```python
from build123d import *

# Parameters (mm, degrees)
ESBO_O1_R                                            = 10.7
RESSALTO_EXTRUS_O1_DEPTH                             = 2.05
RESSALTO_EXTRUS_O2_DEPTH                             = 3
ESBO_O4_W                                            = 25
ESBO_O4_H                                            = 7.35
RESSALTO_EXTRUS_O3_DEPTH                             = 10.8
REBAIXO_PARA_SHCS_M2_51_D                            = 2.9
REBAIXO_PARA_SHCS_M2_51_CBORE_D                      = 5.5
REBAIXO_PARA_SHCS_M2_51_CBORE_DEPTH                  = 10
REBAIXO_PARA_PARAFUSO_COM_CABE_A_REDONDA_D           = 2.4
REBAIXO_PARA_PARAFUSO_COM_CABE_A_REDONDA_CBORE_D     = 4.4
REBAIXO_PARA_PARAFUSO_COM_CABE_A_REDONDA_CBORE_DEPTH = 3.5
PADR_OCIRCULAR1_COUNT                                = 4
NERVURA1_REACH                                       = 67.842
ESBO_O5_WALL_W                                       = 144.857085312
ESBO_O5_WALL_H                                       = 15
CORTE_EXTRUS_O1_REACH                                = 68.053
ESBO_O6_W                                            = 8.93885445
ESBO_O6_H                                            = 8
CORTE_EXTRUS_O2_REACH                                = 68.474
ESBO_O7_R                                            = 3
FILETE1_R                                            = 2


with BuildPart() as part:
    # Esboço1 → Ressalto-extrusão1 (new body)
    with BuildSketch(Plane(origin=(0, 0, 0), x_dir=(-1, 0, 0), z_dir=(0, 0, -1))):
        Circle(ESBO_O1_R)
    extrude(amount=RESSALTO_EXTRUS_O1_DEPTH)

    # Esboço2 → Ressalto-extrusão2 (add)
    with BuildSketch(Plane(origin=(0, 0, -2.05), x_dir=(-1, 0, 0), z_dir=(0, 0, -1))):
        with BuildLine():
            Line((-12.5, 64.388275999), (12.5, 64.388275999))
            Line((12.5, 64.388275999), (12.5, 0))
            ThreePointArc((12.5, 0), (0, -12.5), (-12.5, 0))
            Line((-12.5, 0), (-12.5, 64.388275999))
        make_face()
    extrude(amount=RESSALTO_EXTRUS_O2_DEPTH)

    # Esboço4 → Ressalto-extrusão3 (add)
    with BuildSketch(Plane(origin=(0, 0, -5.05), x_dir=(-1, 0, 0), z_dir=(0, 0, -1))):
        with Locations((0, 60.713275999)):
            Rectangle(ESBO_O4_W, ESBO_O4_H)
    extrude(amount=-RESSALTO_EXTRUS_O3_DEPTH)

    # Rebaixo para SHCS M2.51 (through all)
    with Locations(Plane(origin=(0, 0, -5.05), x_dir=(-1, 0, 0), z_dir=(0, 0, -1))):
        with Locations((-8.5, 61.838275999), (8.5, 61.838275999)):
            CounterBoreHole(REBAIXO_PARA_SHCS_M2_51_D / 2, REBAIXO_PARA_SHCS_M2_51_CBORE_D / 2, REBAIXO_PARA_SHCS_M2_51_CBORE_DEPTH)

    # Rebaixo para parafuso com cabeça redonda de M21 (through all)
    with Locations(Plane(origin=(0, 0, -5.05), x_dir=(-1, 0, 0), z_dir=(0, 0, -1))):
        with Locations((-5.624741587, 5.688785642)):
            rebaixo_para_parafuso_com_cabe_a_redonda = CounterBoreHole(REBAIXO_PARA_PARAFUSO_COM_CABE_A_REDONDA_D / 2, REBAIXO_PARA_PARAFUSO_COM_CABE_A_REDONDA_CBORE_D / 2, REBAIXO_PARA_PARAFUSO_COM_CABE_A_REDONDA_CBORE_DEPTH)

    # PadrãoCircular1: Rebaixo para parafuso com cabeça redonda de M21 ×4 about axis
    padr_ocircular1_axis = Axis((0, 0, 0), (0, 0, 1))
    for i in range(1, PADR_OCIRCULAR1_COUNT):
        add(rebaixo_para_parafuso_com_cabe_a_redonda.rotate(padr_ocircular1_axis, i * 360 / PADR_OCIRCULAR1_COUNT), mode=Mode.SUBTRACT)

    # Esboço5 wall → Nervura1 (add, up to next)
    with BuildSketch(Plane(origin=(0, 53.038275999, 1.85), x_dir=(0, -0.71600013962, -0.69810013613), z_dir=(0, 0.69810013613, -0.71600013962)), mode=Mode.PRIVATE) as nervura1_sk1:
        Rectangle(ESBO_O5_WALL_W, ESBO_O5_WALL_H)
    nervura1_tool1 = extrude(nervura1_sk1.sketch, amount=NERVURA1_REACH, mode=Mode.PRIVATE) - part.part
    add(nervura1_tool1.solids().sort_by_distance((0, 53.038275999, 1.85))[0])

    # Esboço6 → Corte-extrusão1 (cut, up to next)
    with BuildSketch(Plane.XY.offset(-2.05), mode=Mode.PRIVATE) as corte_extrus_o1_sk1:
        with Locations((-0.067802218, 53.038275999)):
            Rectangle(ESBO_O6_W, ESBO_O6_H)
    corte_extrus_o1_tool1 = extrude(corte_extrus_o1_sk1.sketch, amount=CORTE_EXTRUS_O1_REACH, mode=Mode.PRIVATE) & part.part
    add(corte_extrus_o1_tool1.solids().sort_by_distance((-0.067802, 53.038276, -2.05))[0], mode=Mode.SUBTRACT)

    # Esboço7 → Corte-extrusão2 (cut, up to next)
    with BuildSketch(Plane(origin=(0, 0, -5.05), x_dir=(-1, 0, 0), z_dir=(0, 0, -1)), mode=Mode.PRIVATE) as corte_extrus_o2_sk1:
        Circle(ESBO_O7_R)
    corte_extrus_o2_tool1 = extrude(corte_extrus_o2_sk1.sketch, amount=-CORTE_EXTRUS_O2_REACH, mode=Mode.PRIVATE) & part.part
    add(corte_extrus_o2_tool1.solids().sort_by_distance((0, 0, -5.05))[0], mode=Mode.SUBTRACT)

    # Filete1
    filete1_edges = [part.edges().sort_by_distance(p)[0] for p in [
        (10.7, 0, -2.05),
    ]]
    fillet(filete1_edges, radius=FILETE1_R - 0.0001)  # a hair under: the kernel refuses the full size


solid = part.part
```
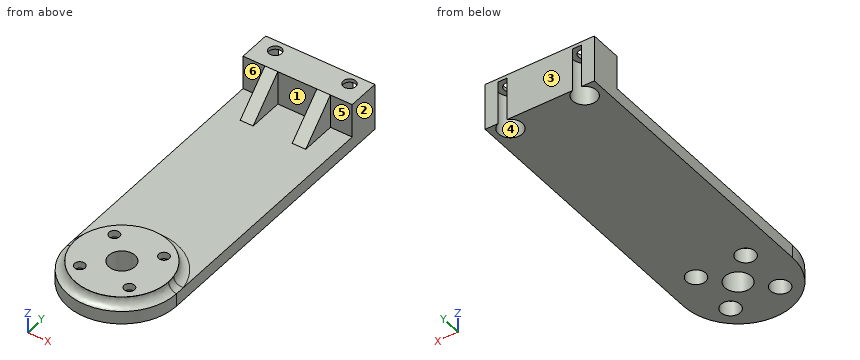
Input: part model. Units: mm. Frame: model coordinates. Face numbers are marked on the shaded views. A direction names the side the tool comes from. Give positions to 0.01 mm unless a question says otherwise; leave off trailing zeros. Order: outer loops, then holes, each group sorted by start corner. A loop starts at its lowest first (then second) coordinate and runs counter-clockwise, first axis right, second up. Notation, with made-up numbers: M 29,36.5 L 65,36.5 A17 ccw 65,49.5 Z; hole C 3,62 d7. An arc over 180 degrees is marked long. One line per question, with ' | ' between items.
1) Access query for the marked faces 4, 5 and 6. Directions: +Z, -Z, +X, -X, +Y, -Y. A direction counts if a zero-diameter tool reaches every point of the face in a straight line with its end or side. Return the directions, or none.
Filled in:
face 4: -Z | face 5: +Z, +X | face 6: +Z, -X
2) Contact query for flat-ended pins moving along their axis: P1, Ø1.3, axis at x = 5.5, y = -5, coming from the -Z side; P2, Ø2.5, axis at x = -8.5, y = 61.84, coming from the +Z side; P3, Ø7.5, axis at x = -3.5, y = 41.5, coming from the +Z side; P4, Ø1.5, axis at y = 6.5, z = -0.5, coming from the +X side. Output: stop coordinate, or through.
Filled in:
P1: stops at z = -1.55 | P2: passes through | P3: stops at z = -2.05 | P4: stops at x = 9.19
3) Ray query, L1, parallel to Z at x = 1, y = 19; L2, parallel to Y at x = 8, z = -1; L3, parallel to Y at x = -3.25, z = 1.75. Return the intervals inside material, ascending.
Filled in:
L1: z = -5.05 to -2.05 | L2: y = -7.45 to 7.46, 57.04 to 59.13 | L3: y = 57.04 to 64.39
4) Draft query along Y for the marked faces 1, 2 and 3. Return one class per face: pulls with the +Y half, pulls with the -Y half, needs draft (parallel to the pull), parting line crosses it, or undercut.
Filled in:
face 1: undercut | face 2: needs draft | face 3: pulls with the +Y half
5) Section B-B on y = 14. Output: boundary loops of the cut face in (x, z).
Filled in:
outline: M -12.5,-5.05 L 12.5,-5.05 L 12.5,-2.05 L -12.5,-2.05 Z
6) Section A-A on z = -0.75. State how many separate pieces and enclosed holes the cut face has, and give its area (3 significant figures).
Filled in:
separate pieces: 2 | enclosed holes: 5 | area: 499 mm2
7) Section C-C on z = 3. Output: boundary loops of the cut face in (x, y).
Filled in:
outline: M -12.5,57.04 L -7.5,57.04 L -7.5,54.22 L -4.54,54.22 L -4.54,57.04 L 4.4,57.04 L 4.4,54.22 L 7.5,54.22 L 7.5,57.04 L 12.5,57.04 L 12.5,64.39 L 9.53,64.39 A2.75 cw long 7.47,64.39 L -7.47,64.39 A2.75 cw long -9.53,64.39 L -12.5,64.39 Z
